Read the model definition and answer for the solid it produces. Units are mm, in the model's axes. A direction names the side the tool comes from. Coordinates: 2 decimals unless noted, no trailing zeros. Loops run counter-clockwise (first coordinate to the right, second up) from the corner with the lowest first, then second, coordinate; pieces in that order, holes last. Notation, with made-up numbers: (66, 87) -> (97, 87) arc R6 cw to (97, 94) -> close; hole circle Ø2 at (19, 2). An arc over 180 degrees is marked (long way). Answer in a Markdown table with one row per item.
```python
from build123d import *

# Parameters (mm, degrees)
F1_DEPTH = 12.7
F2_R     = 6.35
F3_R     = 1.27


with BuildPart() as f1:
    # F0 (on Top) → F1 (new body)
    with BuildSketch(Plane.XY):
        with BuildLine():
            Line((34.29, 31.75), (-34.29, 31.75))
            ThreePointArc((-34.29, 31.75), (-41.474205, 28.774205), (-44.45, 21.59))
            Line((-44.45, 21.59), (-44.45, -21.59))
            ThreePointArc((-44.45, -21.59), (-41.474205, -28.774205), (-34.29, -31.75))
            Line((-34.29, -31.75), (34.29, -31.75))
            ThreePointArc((34.29, -31.75), (41.474205, -28.774205), (44.45, -21.59))
            Line((44.45, -21.59), (44.45, 21.59))
            ThreePointArc((44.45, 21.59), (41.474205, 28.774205), (34.29, 31.75))
        make_face()
        with BuildLine():
            ThreePointArc((34.925, -12.065), (31.949205, -19.249205), (24.765, -22.225))
            Line((24.765, -22.225), (-24.765, -22.225))
            ThreePointArc((-24.765, -22.225), (-31.949205, -19.249205), (-34.925, -12.065))
            Line((-34.925, -12.065), (-34.925, 12.065))
            ThreePointArc((-34.925, 12.065), (-31.949205, 19.249205), (-24.765, 22.225))
            Line((-24.765, 22.225), (24.765, 22.225))
            ThreePointArc((24.765, 22.225), (31.949205, 19.249205), (34.925, 12.065))
            Line((34.925, 12.065), (34.925, -12.065))
        make_face(mode=Mode.SUBTRACT)
    extrude(amount=F1_DEPTH)

    # F2
    f2_edges = [f1.edges().sort_by_distance(p)[0] for p in [
        (-41.474205, -28.774205, 0),
    ]]
    fillet(f2_edges, radius=F2_R)

    # F3
    f3_edges = [f1.edges().sort_by_distance(p)[0] for p in [
        (0, -22.225, 0),
        (-31.949205, -19.249205, 0),
        (-34.925, 0, 0),
        (-31.949205, 19.249205, 0),
        (0, 22.225, 0),
        (31.949205, 19.249205, 0),
        (34.925, 0, 0),
        (31.949205, -19.249205, 0),
    ]]
    fillet(f3_edges, radius=F3_R)


solid = f1.part
```
1. A cutting plane is placed at A-A on y = -2. Give the vertices of the cut face in (x, z) (3 decimals).
A:
| item | result |
|---|---|
| outline | (-44.45, 6.35) arc R6.35 ccw to (-38.1, 0) -> (-36.195, 0) arc R1.27 ccw to (-34.925, 1.27) -> (-34.925, 12.7) -> (-44.45, 12.7) -> close; (34.925, 1.27) arc R1.27 ccw to (36.195, 0) -> (38.1, 0) arc R6.35 ccw to (44.45, 6.35) -> (44.45, 12.7) -> (34.925, 12.7) -> close |
2. A cutting plane is placed at C-C on x = -12. Give the vertices of the cut face in (y, z) (3 decimals), and give its area (3 significant figures).
A:
| item | result |
|---|---|
| outline | (-31.75, 6.35) arc R6.35 ccw to (-25.4, 0) -> (-23.495, 0) arc R1.27 ccw to (-22.225, 1.27) -> (-22.225, 12.7) -> (-31.75, 12.7) -> close; (22.225, 1.27) arc R1.27 ccw to (23.495, 0) -> (25.4, 0) arc R6.35 ccw to (31.75, 6.35) -> (31.75, 12.7) -> (22.225, 12.7) -> close |
| area | 224 mm2 |
3. A tool of negligible diameter and unlimited length cuts with its end or side. For faces 1 (the cylindrical face through (-41.395, 28.853, 9.481)), 2 (the flat face through (34.925, 0, 7)), from which of +Z, -Z, +X, -X, +Y, -Y can it reach the whole face along a straight path? Write none if from no direction.
A:
| item | result |
|---|---|
| face 1 | +Z, -Z, -X, +Y |
| face 2 | +Z, -Z |
4. Find the intervals of material crossed by probe 1 along Y at (x, z) = (21, 6.5) (3 decimals); probe 2 along X at (y, z) = (-11.5, 10) (3 decimals), in increasing order.
A:
| item | result |
|---|---|
| probe 1 | y = -31.75 to -22.225, 22.225 to 31.75 |
| probe 2 | x = -44.45 to -34.925, 34.925 to 44.45 |
5. A cutting plane is placed at B-B on z = 7.75. Give the vertices of the cut face in (x, y) (3 decimals).
A:
| item | result |
|---|---|
| outline | (-44.45, -21.59) arc R10.16 ccw to (-34.29, -31.75) -> (34.29, -31.75) arc R10.16 ccw to (44.45, -21.59) -> (44.45, 21.59) arc R10.16 ccw to (34.29, 31.75) -> (-34.29, 31.75) arc R10.16 ccw to (-44.45, 21.59) -> close; hole (-34.925, -12.065) arc R10.16 ccw to (-24.765, -22.225) -> (24.765, -22.225) arc R10.16 ccw to (34.925, -12.065) -> (34.925, 12.065) arc R10.16 ccw to (24.765, 22.225) -> (-24.765, 22.225) arc R10.16 ccw to (-34.925, 12.065) -> close |
6. Given pin 1 Ø2 at (y, z) = (-1.5, 4) entering from +X; pin 2 Ø12 at (x, y) = (-17.5, -11.5) entering from -Z; pin 3 Ø4 at (x, z) = (31, 1.5) entering from -Y, each flat-ended and moving along its own axis, determine where each tip first touches the part or whether it passes through.
A:
| item | result |
|---|---|
| pin 1 | stops at x = 44.3 |
| pin 2 | passes through |
| pin 3 | stops at y = -31.07 |
7. The mould has two halves that part along X. Classify faces 3 (the cylindrical face through (32, -19.2, 6.9)), 4 (the flat face through (0, 31.75, 9)), 5 (the cylindrical face through (41.395, -28.853, 9.481)), 6 (the flat face through (0, -22.225, 7)): pulls with the +X half, pulls with the -X half, needs draft (parallel to the pull), parting line crosses it, or undercut.
A:
| item | result |
|---|---|
| face 3 | undercut |
| face 4 | needs draft |
| face 5 | pulls with the +X half |
| face 6 | undercut |
